```python
from build123d import *

# Parameters (mm, degrees)
SKETCH2_W               = 33.180430229
SKETCH2_H               = 19.812
SKETCH2_R               = 4.2291
BOSS_EXTRUDE3_DEPTH     = 12.065
CUT_EXTRUDE5_REACH      = 24.87
SKETCH7_R               = 1.4224
CUT_EXTRUDE8_DEPTH      = 23.86983051
CUT_EXTRUDE8_DEPTH_BACK = 23.86983051
SKETCH8_W               = 12.7
SKETCH8_H               = 0.254


with BuildPart() as part:
    # Sketch2 → Boss-Extrude3 (new, symmetric)
    with BuildSketch(Plane.XY):
        with Locations((0.122984885, 0.000254)):
            Rectangle(SKETCH2_W, SKETCH2_H)
        with Locations(Location((7.4041, 0.000254, 0), (0, 0, 180))):
            Circle(SKETCH2_R, mode=Mode.SUBTRACT)
        Polygon((-11.387230229, 0.000254), (-9.334172672, -3.555746), (-5.228057557, -3.555746), (-3.175, 0.000254), (-5.228057557, 3.556254), (-9.334172672, 3.556254), align=None, mode=Mode.SUBTRACT)
    extrude(amount=BOSS_EXTRUDE3_DEPTH, both=True)

    # Sketch7 → Cut-Extrude5 (cut, up to next)
    with BuildSketch(Plane(origin=(0, 0, 0), x_dir=(1, 0, 0), z_dir=(0, 1, 0)), mode=Mode.PRIVATE) as cut_extrude5_sk1:
        with Locations(Location((-7.228125784, -7.62, 0), (0, 0, 270))):
            Circle(SKETCH7_R)
    cut_extrude5_tool1 = extrude(cut_extrude5_sk1.sketch, amount=-CUT_EXTRUDE5_REACH, mode=Mode.PRIVATE) & part.part
    # Sketch7 → Cut-Extrude5 (cut, up to next)
    with BuildSketch(Plane(origin=(0, 0, 0), x_dir=(1, 0, 0), z_dir=(0, 1, 0)), mode=Mode.PRIVATE) as cut_extrude5_sk2:
        with Locations(Location((-7.228125784, 7.62, 0), (0, 0, 270))):
            Circle(SKETCH7_R)
    cut_extrude5_tool2 = extrude(cut_extrude5_sk2.sketch, amount=-CUT_EXTRUDE5_REACH, mode=Mode.PRIVATE) & part.part
    add(cut_extrude5_tool1.solids().sort_by_distance((-7.228126, 0, 7.62))[0], mode=Mode.SUBTRACT)
    add(cut_extrude5_tool2.solids().sort_by_distance((-7.228126, 0, -7.62))[0], mode=Mode.SUBTRACT)

    # Sketch8 → Cut-Extrude8 (cut, two sides: drawn at the far end of the back side and taken through both)
    with BuildSketch(Plane.XY.offset(-CUT_EXTRUDE8_DEPTH_BACK)):
        with Locations((13.86896495, -0.381)):
            Rectangle(SKETCH8_W, SKETCH8_H)
    extrude(amount=CUT_EXTRUDE8_DEPTH + CUT_EXTRUDE8_DEPTH_BACK, mode=Mode.SUBTRACT)


solid = part.part
```
Verification items for the finished model (mm, model axes). A direction names the side the tool comes from. Give positions to 0.01 mm unless a question says otherwise; leave off trailing zeros. Order: outer loops, then holes, each group sorted by start corner. A loop starts at its lowest first (then second) coordinate and runs counter-clockwise, first axis right, second up. Notation, with made-up numbers: (55, -27) -> (90, -27) arc R29 cw to (90, -6) -> close; hole circle Ø9 at (35.5, -2.75). An arc over 180 degrees is marked (long way). One line per item, written item: value.
(1) Draft check along X on faces 1 (the face through (16.713, -5, 0)), 2 (the face through (0, 0, 12.065)), 3 (the face through (-4.187, 1.753, 0.169)). Enter one of: pulls with the +X half, pulls with the -X half, needs draft (parallel to the pull), parting line crosses it, or undercut.
Final values:
face 1: pulls with the +X half
face 2: needs draft
face 3: undercut
(2) Sectioned sample at B-B on y = -7.75. Record the cut outline in (x, z) (3 decimals).
Final values:
outline: (-16.467, -12.065) -> (16.713, -12.065) -> (16.713, 12.065) -> (-16.467, 12.065) -> close; hole circle Ø2.845 at (-7.228, -7.62); hole circle Ø2.845 at (-7.228, 7.62)
(3) Sectioned sample at A-A on z = 0. Record the cut outline in (x, y) (3 decimals).
Final values:
outline: (-16.467, -9.906) -> (16.713, -9.906) -> (16.713, -0.508) -> (11.603, -0.508) arc R4.229 cw (long way) to (11.626, -0.254) -> (16.713, -0.254) -> (16.713, 9.906) -> (-16.467, 9.906) -> close; hole (-11.387, 0) -> (-9.334, -3.556) -> (-5.228, -3.556) -> (-3.175, 0) -> (-5.228, 3.556) -> (-9.334, 3.556) -> close
(4) Sectioned sample at C-C on y = -1. Record the cut outline in (x, z) (1 decimal), then the cut area to 3 significant figures.
Final values:
outline: (-16.5, -12.1) -> (-10.8, -12.1) -> (-10.8, 12.1) -> (-16.5, 12.1) -> close; (-3.8, -12.1) -> (3.3, -12.1) -> (3.3, 12.1) -> (-3.8, 12.1) -> close; (11.5, -12.1) -> (16.7, -12.1) -> (16.7, 12.1) -> (11.5, 12.1) -> close
area: 432 mm^2
(5) Sectioned sample at D-D on z = 7.62. Record the cut outline in (x, y) (3 decimals), then the cut area to 3 significant figures.
Final values:
outline: (-16.467, -9.906) -> (-8.651, -9.906) -> (-8.651, -3.556) -> (-9.334, -3.556) -> (-11.387, 0) -> (-9.334, 3.556) -> (-5.228, 3.556) -> (-3.175, 0) -> (-5.228, -3.556) -> (-5.806, -3.556) -> (-5.806, -9.906) -> (16.713, -9.906) -> (16.713, -0.508) -> (11.603, -0.508) arc R4.229 cw (long way) to (11.626, -0.254) -> (16.713, -0.254) -> (16.713, 9.906) -> (-16.467, 9.906) -> close
area: 538 mm^2
(6) Scan lines: line 1 along Y through (x, z) = (13, -9.25); line 2 along Z through (x, y) = (-8, -6.25) (3 decimals); line 3 along X through (y, z) = (-7.75, -7.62). Record each from-to range of solid material in increasing order. Write a range as [from, to].
Final values:
line 1: [-9.91, -0.51], [-0.25, 9.91]
line 2: [-12.065, -8.815], [-6.425, 6.425], [8.815, 12.065]
line 3: [-16.47, -8.65], [-5.81, 16.71]
(7) Tool access check on faces 4 (the face through (-6.029, -6.686, 8.385)), 5 (the face through (14, -0.254, 0)), 6 (the face through (0, 9.906, 0)), 7 (the face through (-4.216, -1.803, 0.169)). Record the directions out of +Z, -Z, +X, -X, +Y, -Y that give a thin tool (end or side, any length) a straight path to the whole face; none if there is none.
Final values:
face 4: -Y
face 5: +Z, -Z, +X
face 6: +Z, -Z, +X, -X, +Y
face 7: +Z, -Z
